Can you work these out from the model? Positions are in its coordinate system, mm. Face numbers are marked on the shaded views. Coordinates: 2 decimals unless noted, no trailing zeros. Loops run counter-clockwise (first coordinate to the right, second up) from the corner with the lowest first, then second, coordinate; pieces in that order, holes last. Notation, with made-up numbers: (7.5, 86) -> (48.5, 86) arc R22 cw to (48.5, 102) -> close; hole circle Ø4 at (36, -24.5). An arc over 180 degrees is marked (long way). Use one line per item in the form item = value. Start each with the question number.
(1) Imagine slicing it at A-A (x = 0). List the corners of the cut face in (y, z) for me, plus the area to 3 significant figures.
(2) I need wall thicknesses on line 1 (X direction, y = -80, z = 0); line 2 (X direction, y = -36.5, z = -7.5). Which ranges of each line are inside material? Lowest first, please. Write a range as [from, to].
(3) Imagine slicing it at B-B (z = 23). List the corners of the cut face in (x, y) for me, plus the area to 3 significant figures.
(4) I'm going to push flat-ended pins straight in: pin 1 (2.5 mm diameter, centred on x = -28, y = -120.5, fed in from +Z); pin 2 (1.4 mm diameter, centred on x = -27, z = -1, fed in from +Y); pin 3 (4 mm diameter, centred on x = -29, y = -119.5, fed in from -Z); pin 4 (12 mm diameter, centred on x = 18, z = 6, fed in from +Y). Where does each tip first touch, or does it pass through?
(5) Thinking about a two-plate mould opening in Z: for the marked faces 1 and 2, which applies, released by +Z, released by -Z, zero draft, split by the parting line, or undercut?
(6) Imagine slicing it at C-C (y = -140.5). List the corners of the cut face in (x, z) for me, plus the area to 3 significant figures.
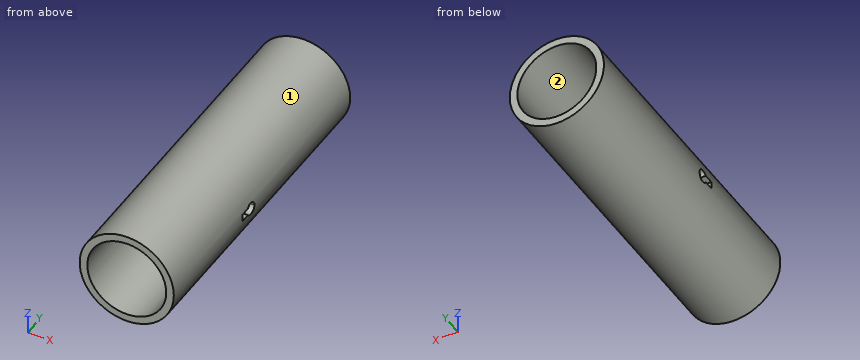
```python
from build123d import *

# Parameters (mm, degrees)
F0_R          = 30.2895
F1_DEPTH      = 203.2
F2_R          = 25.4
F3_DEPTH      = 203.201
F5_DEPTH      = 30.2905
F5_DEPTH_BACK = 30.2905


with BuildPart() as f1:
    # F0 (on Front) → F1 (new body)
    with BuildSketch(Plane.XZ):
        Circle(F0_R)
    extrude(amount=F1_DEPTH)

    # F2 (on face) → F3 (cut, through all)
    with BuildSketch(Plane.XZ.offset(203.2)):
        Circle(F2_R)
    extrude(amount=-F3_DEPTH, mode=Mode.SUBTRACT)

    # F4 (on Right) → F5 (cut, two sides)
    with BuildSketch(Plane.YZ) as f5_sk:
        with BuildLine():
            ThreePointArc((-117.7401898741, -2.1636057012), (-113.1741304801, -3.904934548), (-110.236, 0))
            ThreePointArc((-110.236, 0), (-113.0325941755, 3.8613182304), (-117.5734894076, 2.4083942988))
            Line((-117.5734894076, 2.4083942988), (-117.5734894076, -2.1636057012))
            Line((-117.5734894076, -2.1636057012), (-117.7401898741, -2.1636057012))
        make_face()
        with BuildLine():
            Line((-117.5734894076, -2.1636057012), (-117.5734894076, 2.4083942988))
            ThreePointArc((-117.5734894076, 2.4083942988), (-118.3613013154, 0.1480797953), (-117.7401898741, -2.1636057012))
            Line((-117.7401898741, -2.1636057012), (-117.5734894076, -2.1636057012))
        make_face()
        with BuildLine():
            ThreePointArc((-117.7401898741, -2.1636057012), (-118.3613013154, 0.1480797953), (-117.5734894076, 2.4083942988))
            Line((-117.5734894076, 2.4083942988), (-123.9234894076, 2.4083942988))
            Line((-123.9234894076, 2.4083942988), (-123.9234894076, -2.1636057012))
            Line((-123.9234894076, -2.1636057012), (-117.7401898741, -2.1636057012))
        make_face()
    extrude(amount=-F5_DEPTH, mode=Mode.SUBTRACT)
    extrude(f5_sk.sketch, amount=F5_DEPTH_BACK, mode=Mode.SUBTRACT)


solid = f1.part
```
Worked out:
q1.outline = (-203.2, -30.29) -> (0, -30.29) -> (0, -25.4) -> (-203.2, -25.4) -> close; (-203.2, 25.4) -> (0, 25.4) -> (0, 30.29) -> (-203.2, 30.29) -> close
q1.area = 1,990 mm2
q2.line_1 = [-30.29, -25.4], [25.4, 30.29]
q2.line_2 = [-29.35, -24.27], [24.27, 29.35]
q3.outline = (-19.71, -203.2) -> (-10.78, -203.2) -> (-10.78, 0) -> (-19.71, 0) -> close; (10.78, -203.2) -> (19.71, -203.2) -> (19.71, 0) -> (10.78, 0) -> close
q3.area = 3,630 mm2
q4.pin_1 = 14.21
q4.pin_2 = 0
q4.pin_3 = -13.73
q4.pin_4 = through
q5.face_1 = split by the parting line
q5.face_2 = undercut
q6.outline = circle Ø60.58 at (0, 0); hole circle Ø50.8 at (0, 0)
q6.area = 855 mm2
